Part print with two shaded views. Sizes in mm from the minimum x, y, z corner. A direction names the side the tool comes from. Coordinates: 2 decimals unless noted, no trailing zeros. Loops run counter-clockwise (first coordinate to the right, second up) from the corner with the lowest first, then second, coordinate; pieces in that order, holes last.
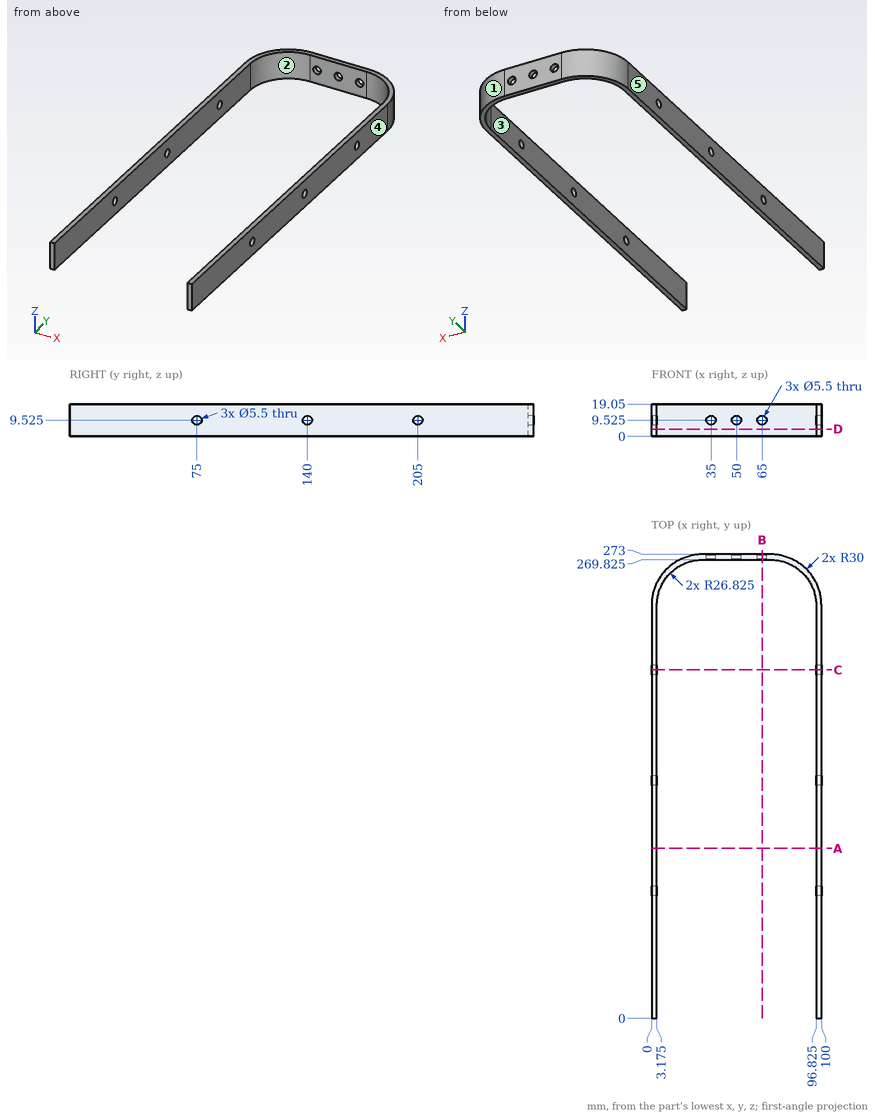
Q1. Mould opens along X. For the marked faces 3, 4 and 5 say: +X half, -X half, draft (parallel to the pull), parting line (faces both ways), or undercut.
Answers:
face 3: undercut
face 4: +X half
face 5: -X half
Q2. Slice it at C-C (y = 205). List the corners of the cut face in (x, z) (3 decimals), and give its area (3 significant figures).
Answers:
outline: (0, 0) - (3.175, 0) - (3.175, 6.775) - (0, 6.775) - close; (0, 12.275) - (3.175, 12.275) - (3.175, 19.05) - (0, 19.05) - close; (96.825, 0) - (100, 0) - (100, 6.775) - (96.825, 6.775) - close; (96.825, 12.275) - (100, 12.275) - (100, 19.05) - (96.825, 19.05) - close
area: 86.0 mm2
Q3. Slice it at D-D (z = 4.25). List the corners of the cut face in (x, y) (3 decimals), and give its area (3 significant figures).
Answers:
outline: (0, 0) - (3.175, 0) - (3.175, 243) arc R26.825 cw to (30, 269.825) - (70, 269.825) arc R26.825 cw to (96.825, 243) - (96.825, 0) - (100, 0) - (100, 243) arc R30 ccw to (70, 273) - (30, 273) arc R30 ccw to (0, 243) - close
area: 1,950 mm2
Q4. Slice it at B-B (x = 65). List the corners of the cut face in (y, z) (3 decimals), and give its area (3 significant figures).
Answers:
outline: (269.825, 0) - (273, 0) - (273, 6.775) - (269.825, 6.775) - close; (269.825, 12.275) - (273, 12.275) - (273, 19.05) - (269.825, 19.05) - close
area: 43.0 mm2
Q5. Which spindle directions (+Z, -Z, +X, -X, +Y, -Y) get a long thin tool onto all of the face, cutting with end or side? Do the marked faces 1 and 2. Say none if no direction does.
Answers:
face 1: +Z, -Z, +X, +Y
face 2: +Z, -Z, -Y
Q6. Slice it at A-A (y = 100). List the corners of the cut face in (x, z) (3 decimals), and give its area (3 significant figures).
Answers:
outline: (0, 0) - (3.175, 0) - (3.175, 19.05) - (0, 19.05) - close; (96.825, 0) - (100, 0) - (100, 19.05) - (96.825, 19.05) - close
area: 121 mm2
Q7. Flat gauge pins, fed straight in: P1, Ø9.5, axis at x = 46.5, z = 10, coming from the -Y side (3 decimals); P2, Ø5, axis at x = 80, z = 7.5, coming from the -Y side; P3, Ø1.5, axis at x = 22.5, z = 11.5, coming from the -Y side. Where does each tip first touch, or does it go through?
Answers:
P1: stops at y = 269.825
P2: stops at y = 266.73
P3: stops at y = 268.52
Q8. Drill centre lines: line 1 (X direction, y = 227, z = 7.5) (3 decimals); line 2 (Z direction, x = 1.3, y = 140) (3 decimals); line 3 (Y direction, x = 69, z = 18.25) (3 decimals). Where is each one in solid material? Low to high.
Answers:
line 1: x = 0 to 3.175, 96.825 to 100
line 2: z = 0 to 6.775, 12.275 to 19.05
line 3: y = 269.825 to 273
